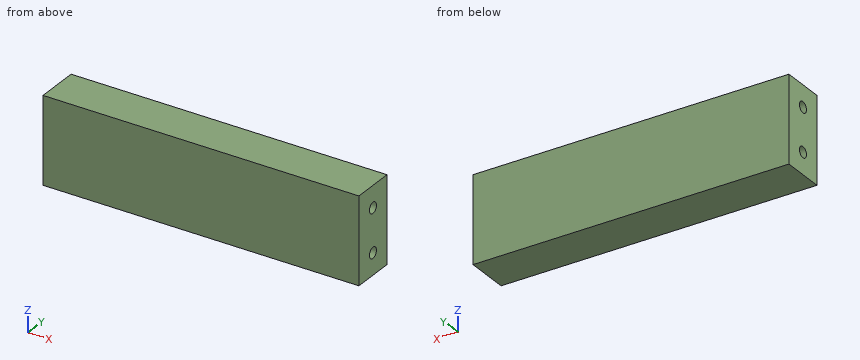
```python
from build123d import *

# Parameters (mm, degrees)
SKETCH_1_W          = 73
SKETCH_1_H          = 20
EXTRUDE_1_DEPTH     = 10
SKETCH_2_R          = 1.25
CUT_EXTRUDE_1_DEPTH = 20


with BuildPart() as part:
    # 草图1 → 凸台-拉伸1 (new body)
    with BuildSketch(Plane(origin=(0, 0, 0), x_dir=(1, 0, 0), z_dir=(0, 1, 0))):
        Rectangle(SKETCH_1_W, SKETCH_1_H)
    extrude(amount=EXTRUDE_1_DEPTH)

    # 草图2 → 切除-拉伸1 (cut)
    with BuildSketch(Plane(origin=(36.5, 0, 0), x_dir=(0, 0, -1), z_dir=(1, 0, 0))):
        with Locations((-5, 5)):
            Circle(SKETCH_2_R)
        with Locations((5, 5)):
            Circle(SKETCH_2_R)
    cut_extrude_1 = extrude(amount=-CUT_EXTRUDE_1_DEPTH, mode=Mode.SUBTRACT)

    # 镜向1: 切除-拉伸1 across plane
    add(cut_extrude_1.mirror(Plane(origin=(0, 0, 0), x_dir=(0, 0, 1), z_dir=(1, 0, 0))), mode=Mode.SUBTRACT)


solid = part.part
```
Build history of the part. All positions in model axes, mm. Coordinates: 2 decimals unless noted, no trailing zeros. Write each loop counter-clockwise with the first axis right and the second up, starting at its lowest first coordinate (ties: lowest second). Pieces come first, ordered by that corner, then holes.
1. Band-saw the part on A-A, the plane z = -5. Give the cut face in (x, y).
Answer block:
outline: (-36.5, 0) - (36.5, 0) - (36.5, 3.75) - (16.5, 3.75) - (16.5, 6.25) - (36.5, 6.25) - (36.5, 10) - (-36.5, 10) - (-36.5, 6.25) - (-16.5, 6.25) - (-16.5, 3.75) - (-36.5, 3.75) - close
2. Drill centre lines: probe 1 along Y at (x, z) = (-23.5, -5); probe 2 along Z at (x, y) = (-24.5, 4.5); probe 3 along X at (y, z) = (5, -6). Where is each one in solid material? Low to high.
Answer block:
probe 1: y = 0 to 3.75, 6.25 to 10
probe 2: z = -10 to -6.15, -3.85 to 3.85, 6.15 to 10
probe 3: x = -16.5 to 16.5
3. Drop flat-ended pins along their axis: pin 1 (1.5 mm diameter, centred on y = 5, z = 5, fed in from +X); pin 2 (2 mm diameter, centred on y = 5, z = -5, fed in from -X). Give the stop position or say it passes through.
Answer block:
pin 1: stops at x = 16.5
pin 2: stops at x = -16.5
4. Band-saw the part on B-B, the plane x = 28. Give the cut face in (y, z).
Answer block:
outline: (0, -10) - (10, -10) - (10, 10) - (0, 10) - close; hole circle Ø2.5 at (5, -5); hole circle Ø2.5 at (5, 5)
5. Band-saw the part on C-C, the plane y = 5. Give the cut face in (x, z).
Answer block:
outline: (-36.5, -10) - (36.5, -10) - (36.5, -6.25) - (16.5, -6.25) - (16.5, -3.75) - (36.5, -3.75) - (36.5, 3.75) - (16.5, 3.75) - (16.5, 6.25) - (36.5, 6.25) - (36.5, 10) - (-36.5, 10) - (-36.5, 6.25) - (-16.5, 6.25) - (-16.5, 3.75) - (-36.5, 3.75) - (-36.5, -3.75) - (-16.5, -3.75) - (-16.5, -6.25) - (-36.5, -6.25) - close
